For this review, take the finished solid that the model builds, in its own axes (mm). A direction names the side the tool comes from. Give positions to 0.01 mm unless a question says otherwise; leave off trailing zeros. Loops run counter-clockwise (first coordinate to the right, second up) from the corner with the lowest first, then second, coordinate; pieces in that order, holes last. Notation, with made-up numbers: (86.5, 60.25) -> (134.5, 60.25) arc R26 ccw to (134.5, 80.25) -> close; hole circle Ø9 at (82, 5). An arc over 180 degrees is marked (long way). Answer as CSV lines item,"result". Start each with the question number.
Item 1: For L1, parallel to Z at x = 3, y = 23.25; L2, parallel to Y at x = -1.75, z = 1.95; L3, parallel to Y at x = 1.75, z = 0.3, list the stretches that pass through material, from the lowest coordinate up. Write a range as from..to.
Item 2: Clearance check with a flat-ended pin moving along its axis: P1, Ø0.5, axis at y = 12.5, z = 1.5, coming from the -X side. State where the tip first meets the part, or that it passes through.
Item 3: Add section B-B on x = -5.5. State the section outline as (y, z) points.
Item 4: Add section C-C on z = 1.9. State the section outline as (x, y) points.
Item 5: Add section A-A on y = 18.75. State the section outline as (x, z) points.
Item 6: Machinability: for faces 1 (the face through (0, 19.7, 2)), 2 (the face through (0, 0.452, 2)), 3 (the face through (-6.261, 10, 2)), which of the approach directions +Z, -Z, +X, -X, +Y, -Y give a long, thin tool a straight path to every point of the face, cutting with its end or side? Answer none if there is none.
```python
from build123d import *

# Parameters (mm, degrees)
F0_W     = 13.4
F0_H     = 25.8
F1_DEPTH = 0.8
F2_R     = 0.4
F3_DEPTH = 25
F4_W     = 12.522456
F4_H     = 19.248359
F5_DEPTH = 1.6


with BuildPart() as f1:
    # F0 (on Top) → F1 (new body)
    with BuildSketch(Plane.XY):
        with Locations((0, 12.9)):
            Rectangle(F0_W, F0_H)
    extrude(amount=F1_DEPTH)

    # F2 (on face) → F3 (cut)
    with BuildSketch(Plane.XY.offset(0.8)):
        with Locations((-6.7, 2.8)):
            Circle(F2_R)
        with Locations((-6.7, 4)):
            Circle(F2_R)
        with Locations((-6.7, 5.2)):
            Circle(F2_R)
        with Locations((-6.7, 6.4)):
            Circle(F2_R)
        with Locations((-6.7, 7.6)):
            Circle(F2_R)
        with Locations((-6.7, 8.8)):
            Circle(F2_R)
        with Locations((-6.7, 10)):
            Circle(F2_R)
        with Locations((-6.7, 11.2)):
            Circle(F2_R)
        with Locations((-6.7, 12.4)):
            Circle(F2_R)
        with Locations((-6.7, 13.6)):
            Circle(F2_R)
        with Locations((-6.7, 14.8)):
            Circle(F2_R)
        with Locations((-6.7, 16)):
            Circle(F2_R)
        with Locations((6.7, 2.8)):
            Circle(F2_R)
        with Locations((6.7, 4)):
            Circle(F2_R)
        with Locations((6.7, 5.2)):
            Circle(F2_R)
        with Locations((6.7, 6.4)):
            Circle(F2_R)
        with Locations((6.7, 7.6)):
            Circle(F2_R)
        with Locations((6.7, 8.8)):
            Circle(F2_R)
        with Locations((6.7, 10)):
            Circle(F2_R)
        with Locations((6.7, 11.2)):
            Circle(F2_R)
        with Locations((6.7, 12.4)):
            Circle(F2_R)
        with Locations((6.7, 13.6)):
            Circle(F2_R)
        with Locations((6.7, 14.8)):
            Circle(F2_R)
        with Locations((6.7, 16)):
            Circle(F2_R)
        with Locations((-4.1, 0)):
            Circle(F2_R)
        with Locations((-3.1, 0)):
            Circle(F2_R)
        with Locations((-1.8, 0)):
            Circle(F2_R)
        with Locations((-0.6, 0)):
            Circle(F2_R)
        with Locations((0.6, 0)):
            Circle(F2_R)
        with Locations((1.8, 0)):
            Circle(F2_R)
        with Locations((3.1, 0)):
            Circle(F2_R)
        with Locations((4.1, 0)):
            Circle(F2_R)
    extrude(amount=-F3_DEPTH, mode=Mode.SUBTRACT)

    # F4 (on face) → F5 (join)
    with BuildSketch(Plane.XY.offset(0.8)):
        with Locations((0, 10.07582)):
            Rectangle(F4_W, F4_H)
    extrude(amount=F5_DEPTH)


solid = f1.part
```
Computed values:
1,L1,"0..0.8"
1,L2,"0.45..19.7"
1,L3,"0.4..25.8"
2,P1,"x = -6.26"
3,outline,"(0, 0) -> (25.8, 0) -> (25.8, 0.8) -> (19.7, 0.8) -> (19.7, 2.4) -> (0.45, 2.4) -> (0.45, 0.8) -> (0, 0.8) -> close"
4,outline,"(-6.26, 0.45) -> (6.26, 0.45) -> (6.26, 19.7) -> (-6.26, 19.7) -> close"
5,outline,"(-6.7, 0) -> (6.7, 0) -> (6.7, 0.8) -> (6.26, 0.8) -> (6.26, 2.4) -> (-6.26, 2.4) -> (-6.26, 0.8) -> (-6.7, 0.8) -> close"
6,face 1,"+Z, +X, -X, +Y"
6,face 2,"+Z, +X, -X, -Y"
6,face 3,"+Z, -X, +Y, -Y"
